The listing builds one solid part. Answer for the finished solid, in the listing's coordinates (mm). A direction names the side the tool comes from. Coordinates: 2 decimals unless noted, no trailing zeros. Write each loop counter-clockwise with the first axis right and the second up, starting at its lowest first coordinate (ties: lowest second). Pieces come first, ordered by that corner, then holes.
from build123d import *

# Parameters (mm, degrees)
SKETCH1_W           = 105
SKETCH1_H           = 200
BOSS_EXTRUDE1_DEPTH = 40
SKETCH2_W           = 95
SKETCH2_H           = 190
CUT_EXTRUDE1_DEPTH  = 35
FILLET1_R           = 10
SKETCH3_R           = 1.6
CUT_EXTRUDE2_DEPTH  = 35
BOSS_EXTRUDE2_DEPTH = 10
SKETCH6_R           = 2.5
CUT_EXTRUDE3_DEPTH  = 10
SKETCH7_R           = 13
SKETCH7_R_2         = 5
CUT_EXTRUDE5_DEPTH  = 7
SKETCH9_W           = 10
SKETCH9_H           = 4.718519443
CUT_EXTRUDE8_DEPTH  = 7
SKETCH10_W          = 11.630652226
SKETCH10_H          = 3.85031924
CUT_EXTRUDE11_DEPTH = 7
SKETCH11_W          = 2
SKETCH11_H          = 11.091513068
SKETCH11_H_2        = 11.156323384
CUT_EXTRUDE12_DEPTH = 7
CUT_EXTRUDE13_DEPTH = 7
SKETCH13_R          = 3.5
CUT_EXTRUDE14_DEPTH = 7


with BuildPart() as part:
    # Sketch1 → Boss-Extrude1 (new body)
    with BuildSketch(Plane.XY):
        with Locations((52.5, 100)):
            Rectangle(SKETCH1_W, SKETCH1_H)
    extrude(amount=BOSS_EXTRUDE1_DEPTH)

    # Sketch2 → Cut-Extrude1 (cut)
    with BuildSketch(Plane.XY.offset(40)):
        with Locations((52.5, 100)):
            Rectangle(SKETCH2_W, SKETCH2_H)
    extrude(amount=-CUT_EXTRUDE1_DEPTH, mode=Mode.SUBTRACT)

    # Fillet1
    fillet1_edges = [part.edges().sort_by_distance(p)[0] for p in [
        (5, 195, 22.5),
        (100, 195, 22.5),
        (100, 5, 22.5),
        (5, 5, 22.5),
        (0, 200, 20),
        (105, 200, 20),
        (105, 0, 20),
        (0, 0, 20),
    ]]
    fillet(fillet1_edges, radius=FILLET1_R)

    # Sketch3 → Cut-Extrude2 (cut)
    with BuildSketch(Plane.XY.offset(40)):
        with Locations((6, 194)):
            Circle(SKETCH3_R)
        with Locations((99, 194)):
            Circle(SKETCH3_R)
        with Locations((99, 6)):
            Circle(SKETCH3_R)
        with Locations((6, 6)):
            Circle(SKETCH3_R)
    extrude(amount=-CUT_EXTRUDE2_DEPTH, mode=Mode.SUBTRACT)

    # Sketch4 → Boss-Extrude2 (add)
    with BuildSketch(Plane.XY.offset(40)):
        with BuildLine():
            Line((21, 200), (21, 206))
            ThreePointArc((21, 206), (26, 235.142135624), (31, 206))
            Line((31, 206), (31, 200))
            Line((31, 200), (21, 200))
        make_face()
    extrude(amount=-BOSS_EXTRUDE2_DEPTH)

    # Sketch6 → Cut-Extrude3 (cut)
    with BuildSketch(Plane.XY.offset(40)):
        with Locations((26, 220.142135624)):
            Circle(SKETCH6_R)
    extrude(amount=-CUT_EXTRUDE3_DEPTH, mode=Mode.SUBTRACT)

    # Sketch7 → Cut-Extrude5 (cut)
    with BuildSketch(Plane.XY.offset(40)):
        with Locations((26, 220.142135624)):
            Circle(SKETCH7_R)
        with Locations((26, 220.142135624)):
            Circle(SKETCH7_R_2, mode=Mode.SUBTRACT)
    extrude(amount=-CUT_EXTRUDE5_DEPTH, mode=Mode.SUBTRACT)

    # Sketch9 → Cut-Extrude8 (cut)
    with BuildSketch(Plane.XY.offset(40)):
        with Locations((26, 233.858468974)):
            Rectangle(SKETCH9_W, SKETCH9_H)
    extrude(amount=-CUT_EXTRUDE8_DEPTH, mode=Mode.SUBTRACT)

    # Sketch10 → Cut-Extrude11 (cut)
    with BuildSketch(Plane.XY.offset(40)):
        with Locations((25.887552525, 207.506070883)):
            Rectangle(SKETCH10_W, SKETCH10_H)
    extrude(amount=-CUT_EXTRUDE11_DEPTH, mode=Mode.SUBTRACT)

    # Sketch11 → Cut-Extrude12 (cut)
    with BuildSketch(Plane.XY.offset(40)):
        with Locations((24, 200.229066802)):
            Rectangle(SKETCH11_W, SKETCH11_H)
        with Locations((28, 200.296138355)):
            Rectangle(SKETCH11_W, SKETCH11_H_2)
    extrude(amount=-CUT_EXTRUDE12_DEPTH, mode=Mode.SUBTRACT)

    # Sketch12 → Cut-Extrude13 (cut)
    with BuildSketch(Plane(origin=(0, 0, 30), x_dir=(-1, 0, 0), z_dir=(0, 0, -1))):
        with BuildLine():
            ThreePointArc((-18.666666667, 229.640673523), (-26, 232.142135624), (-33.333333333, 229.640673523))
            ThreePointArc((-33.333333333, 229.640673523), (-33.874634475, 225.432705715), (-29.666666667, 224.891404573))
            ThreePointArc((-29.666666667, 224.891404573), (-26, 226.142135624), (-22.333333333, 224.891404573))
            ThreePointArc((-22.333333333, 224.891404573), (-18.125365525, 225.432705715), (-18.666666667, 229.640673523))
        make_face()
        with BuildLine():
            ThreePointArc((-18.666666667, 210.643597725), (-26, 208.142135624), (-33.333333333, 210.643597725))
            ThreePointArc((-33.333333333, 210.643597725), (-33.874634475, 214.851565533), (-29.666666667, 215.392866674))
            ThreePointArc((-29.666666667, 215.392866674), (-26, 214.142135624), (-22.333333333, 215.392866674))
            ThreePointArc((-22.333333333, 215.392866674), (-18.125365525, 214.851565533), (-18.666666667, 210.643597725))
        make_face()
    extrude(amount=-CUT_EXTRUDE13_DEPTH, mode=Mode.SUBTRACT)

    # Sketch13 → Cut-Extrude14 (cut)
    with BuildSketch(Plane(origin=(0, 0, 30), x_dir=(-1, 0, 0), z_dir=(0, 0, -1))):
        with Locations((-17, 220.142135624)):
            Circle(SKETCH13_R)
        with Locations((-35, 220.142135624)):
            Circle(SKETCH13_R)
    extrude(amount=-CUT_EXTRUDE14_DEPTH, mode=Mode.SUBTRACT)


solid = part.part
1. A tool of negligible diameter and unlimited length cuts with its end or side. For faces 1 (the flat face through (5, 99, 23)), 2 (the cylindrical face through (18.166, 214.903, 31.479)), 3 (the flat face through (31, 203, 35)), from which of +Z, -Z, +X, -X, +Y, -Y can it reach the whole face along a straight path? Write none if from no direction.
Results found:
face 1: +Z
face 2: +Z, -Z
face 3: +Z, -Z, +X
2. Flat-ended cylindrical pins translate along their axes: P1, Ø1, axis at x = 44, z = 11, coming from the +Y side; P2, Ø3, axis at x = 6, y = 6, coming from the +Z side; P3, Ø1, axis at x = 22.5, z = 36.5, coming from the +Y side. Find the tip coordinate at first contact, or state that the pin passes through.
Results found:
P1: stops at y = 200
P2: stops at z = 5
P3: stops at y = 224.14
3. For a pull along X with two mould halves and no side action, classify faces 4 (the cylindrical face through (16.781, 231.975, 35.07)), 5 (the cylindrical face through (33.914, 225.485, 31.479)), 6 (the cylindrical face through (101.99, 197.15, 20.28)), 7 (the flat face through (103, 73, 40)) as pulls with the +X half, pulls with the -X half, needs draft (parallel to the pull), parting line crosses it, or undercut.
Results found:
face 4: parting line crosses it
face 5: undercut
face 6: pulls with the +X half
face 7: needs draft
4. Find the intervals of material crossed by L1, parallel to Y at x = 77.5, z = 34; L2, parallel to X at y = 48, z = 32; L3, parallel to Y at x = 17, z = 32, in increasing order.
Results found:
L1: y = 0 to 5, 195 to 200
L2: x = 0 to 5, 100 to 105
L3: y = 0 to 5, 195 to 200, 208.14 to 216.64, 223.64 to 232.14
5. Section A-A on z = 13.5 is taken. Give the vertices of the cut face in (x, y).
Results found:
outline: (0, 10) arc R10 ccw to (10, 0) - (95, 0) arc R10 ccw to (105, 10) - (105, 190) arc R10 ccw to (95, 200) - (10, 200) arc R10 ccw to (0, 190) - close; hole circle Ø3.2 at (6, 6); hole circle Ø3.2 at (6, 194); hole (5, 15) arc R10 ccw to (15, 5) - (90, 5) arc R10 ccw to (100, 15) - (100, 185) arc R10 ccw to (90, 195) - (15, 195) arc R10 ccw to (5, 185) - close; hole circle Ø3.2 at (99, 6); hole circle Ø3.2 at (99, 194)
6. Section C-C on x = 86 is taken. Give the vertices of the cut face in (y, z), then the cut area to 3 significant figures.
Results found:
outline: (0, 0) - (200, 0) - (200, 40) - (195, 40) - (195, 5) - (5, 5) - (5, 40) - (0, 40) - close
area: 1,350 mm2
7. Section B-B on y = 67.5 is taken. Give the vertices of the cut face in (x, z).
Results found:
outline: (0, 0) - (105, 0) - (105, 40) - (100, 40) - (100, 5) - (5, 5) - (5, 40) - (0, 40) - close
